The model under review builds one solid part; all positions refer to its coordinate system, in mm. A direction names the side the tool comes from. Coordinates: 2 decimals unless noted, no trailing zeros. Write each loop counter-clockwise with the first axis right and the second up, starting at its lowest first coordinate (ties: lowest second). Pieces come first, ordered by that corner, then holes. Notation, with made-up numbers: (87.5, 10) - (100.5, 10) arc R14 cw to (100.5, 35) - close; hole circle Ø9 at (-30, 45). An arc over 180 degrees is marked (long way). Put each result on its own line as item: value. Start each with the question number.
Item 1: Consider section B-B on x = -8.5. Give the boundary of the cut face in (y, z), then the cut area to 3 significant figures.
Item 2: Consider section D-D on y = -9. Give the boundary of the cut face in (x, z).
Item 3: For pin 1 (3 mm diameter, centred on y = -7.5, z = -43, fed in from +X); pin 2 (5 mm diameter, centred on y = -5, z = -28.5, fed in from -X); pin 3 (6 mm diameter, centred on y = -2.5, z = -15, fed in from -X), all flat-tipped, find the tip position at first contact; note any pin that passes through.
Item 4: To check wall thickness, follow L1, parallel to Z at x = -0.25, y = -5; L2, parallel to Z at x = 0, y = -3.25; L3, parallel to X at y = -9, z = -45. State the ranges of each line that lie inside material, in increasing order. Write a range as [from, to].
Item 5: Consider section C-C on z = 3. Give the boundary of the cut face in (x, y), then the cut area to 3 significant figures.
Item 6: Machinability: for faces 1 (the face through (12.5, -5, -41)), 2 (the face through (0, -5, -65.612)), 3 (the face through (-12.5, -5, -40)), which of the approach directions +Z, -Z, +X, -X, +Y, -Y give a long, thin tool a straight path to every point of the face, cutting with its end or side? Answer none if there is none.
Item 7: Mouldability with a two-part tool opening along Y and no side actions: class faces 4 (the face through (-0.17, -4.35, -58.54)), 5 (the face through (0, -10, -22)), 6 (the face through (0, 0, -22)), 7 (the face through (-14.985, -4.93, 0.66)) as pulls with the +Y half, pulls with the -Y half, needs draft (parallel to the pull), parting line crosses it, or undercut.
Item 8: Consider section A-A on y = -5. Give the boundary of the cut face in (x, z).
```python
from build123d import *

# Parameters (mm, degrees)
F0_R     = 15
F1_DEPTH = 10
F3_D     = 6


with BuildPart() as f1:
    # F0 (on Front) → F1 (new body)
    with BuildSketch(Plane.XZ):
        with BuildLine():
            ThreePointArc((12.5, -15.612495), (18.027756, -8.660254), (20, 0))
            ThreePointArc((20, 0), (-8.660254, 18.027756), (-12.5, -15.612495))
            Line((-12.5, -15.612495), (12.5, -15.612495))
        make_face()
        Circle(F0_R, mode=Mode.SUBTRACT)
        with BuildLine():
            ThreePointArc((12.5, -15.612495), (0, -20), (-12.5, -15.612495))
            Line((-12.5, -15.612495), (-12.5, -65.612495))
            Line((-12.5, -65.612495), (12.5, -65.612495))
            Line((12.5, -65.612495), (12.5, -15.612495))
        make_face()
        with BuildLine():
            Line((12.5, -15.612495), (-12.5, -15.612495))
            ThreePointArc((-12.5, -15.612495), (0, -20), (12.5, -15.612495))
        make_face()
    extrude(amount=F1_DEPTH)

    # F3 (through all)
    with Locations(Plane.YZ.offset(12.5)):
        with Locations((-5, -55.612495)):
            Hole(F3_D / 2)


solid = f1.part
```
Report:
1. outline: (-10, -65.61) - (0, -65.61) - (0, -12.36) - (-10, -12.36) - close; (-10, 12.36) - (0, 12.36) - (0, 18.1) - (-10, 18.1) - close; hole circle Ø6 at (-5, -55.61)
1. area: 562 mm²
2. outline: (-12.5, -65.61) - (12.5, -65.61) - (12.5, -15.61) arc R20 ccw to (20, 0) arc R20 ccw (long way) to (-12.5, -15.61) - close; hole circle Ø30 at (0, 0)
3. pin 1: x = 12.5
3. pin 2: x = -12.5
3. pin 3: x = -16
4. L1: [-65.61, -58.61], [-52.61, -15], [15, 20]
4. L2: [-65.61, -58.05], [-53.18, -15], [15, 20]
4. L3: [-12.5, 12.5]
5. outline: (-19.77, -10) - (-14.7, -10) - (-14.7, 0) - (-19.77, 0) - close; (14.7, -10) - (19.77, -10) - (19.77, 0) - (14.7, 0) - close
5. area: 102 mm²
6. face 1: -Z, +X, +Y, -Y
6. face 2: -Z, +X, -X, +Y, -Y
6. face 3: -Z, -X, +Y, -Y
7. face 4: undercut
7. face 5: pulls with the -Y half
7. face 6: pulls with the +Y half
7. face 7: needs draft
8. outline: (-12.5, -65.61) - (12.5, -65.61) - (12.5, -58.61) - (-12.5, -58.61) - close; (-12.5, -52.61) - (12.5, -52.61) - (12.5, -15.61) arc R20 ccw to (20, 0) arc R20 ccw (long way) to (-12.5, -15.61) - close; hole circle Ø30 at (0, 0)
